Part model, mm, in its own coordinate system. Face numbers are marked on the shaded views. A direction names the side the tool comes from. Give positions to 0.01 mm unless a question says otherwise; leave off trailing zeros. Write each loop counter-clockwise with the first axis right and the second up, starting at its lowest first coordinate (ties: lowest second). Pieces come first, ordered by that corner, then holes. Notation, with made-up numbers: M -12.75,18.5 L 18.25,18.5 A11 ccw 18.25,39.5 Z; hole C -12,34 d2. An arc over 180 degrees is marked long. Use CSV: the item, a comma, the result in double quotes. Start each with the question number.
1. Band-saw the part on A-A, the plane x = 0. List the corners of the cut face in (y, z).
2. 3-axis set-ups, long thin cutter, end or side, ignore diameter. For the marked faces 1 and 2: which of +Z, -Z, +X, -X, +Y, -Y reach the whole face in a straight line?
3. Band-saw the part on C-C, the plane x = -27. List the corners of the cut face in (y, z).
4. Drill centre lines: line 1 along Z through (x, y) = (17.5, -4); line 2 along Z through (x, y) = (30, -34.5); line 3 along Y through (x, z) = (13, 2.25). Where is each one in solid material? Low to high. Write a range as from..to.
5. Band-saw the part on D-D, the plane y = 18.5. List the corners of the cut face in (x, z), then the cut area to 3 significant figures.
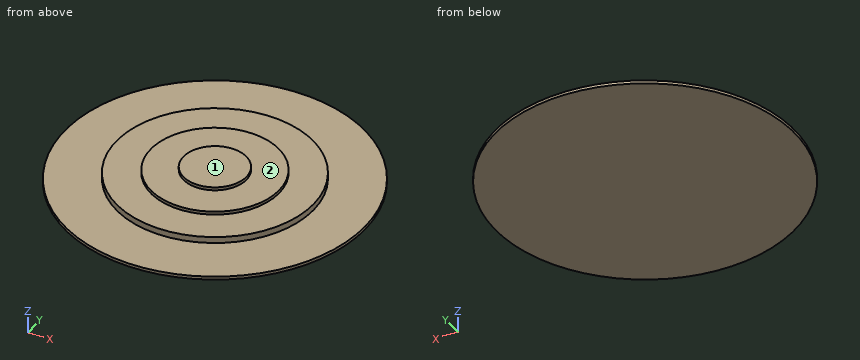
from build123d import *

# Parameters (mm, degrees)
F0_R     = 47.875264
F1_DEPTH = 1
F2_R     = 31.457389
F3_DEPTH = 3
F4_R     = 20.49811
F5_DEPTH = 4
F6_R     = 10.07473
F7_DEPTH = 5


with BuildPart() as f1:
    # F0 (on Top) → F1 (new body)
    with BuildSketch(Plane.XY):
        Circle(F0_R)
    extrude(amount=F1_DEPTH)

    # F2 (on Top) → F3 (join)
    with BuildSketch(Plane.XY):
        Circle(F2_R)
    extrude(amount=F3_DEPTH)

    # F4 (on Top) → F5 (join)
    with BuildSketch(Plane.XY):
        Circle(F4_R)
    extrude(amount=F5_DEPTH)

    # F6 (on Top) → F7 (join)
    with BuildSketch(Plane.XY):
        Circle(F6_R)
    extrude(amount=F7_DEPTH)


solid = f1.part
Output:
1,outline,"M -47.88,0 L 47.88,0 L 47.88,1 L 31.46,1 L 31.46,3 L 20.5,3 L 20.5,4 L 10.07,4 L 10.07,5 L -10.07,5 L -10.07,4 L -20.5,4 L -20.5,3 L -31.46,3 L -31.46,1 L -47.88,1 Z"
2,face 1,"+Z, +X, -X, +Y, -Y"
2,face 2,"+Z"
3,outline,"M -39.54,0 L 39.54,0 L 39.54,1 L 16.14,1 L 16.14,3 L -16.14,3 L -16.14,1 L -39.54,1 Z"
4,line 1,"z = 0..4"
4,line 2,"z = 0..1"
4,line 3,"y = -28.65..28.65"
5,outline,"M -44.16,0 L 44.16,0 L 44.16,1 L 25.44,1 L 25.44,3 L 8.83,3 L 8.83,4 L -8.83,4 L -8.83,3 L -25.44,3 L -25.44,1 L -44.16,1 Z"
5,area,"208 mm²"
